The model under review builds one solid part; all positions refer to its coordinate system, in mm. A direction names the side the tool comes from. Round coordinates to 2 decimals unless told otherwise and drop trailing zeros. Loops run counter-clockwise (first coordinate to the right, second up) from the corner with the lowest first, then second, coordinate; pieces in that order, holes last. Notation, with made-up numbers: (48.25, 25) -> (85.25, 25) arc R27 cw to (85.25, 56) -> close; hole circle Ø10 at (-26, -11.75). An arc over 180 degrees is marked (long way). Return JSON: item names as keys, results as strings. Group by question number.
```python
from build123d import *

# Parameters (mm, degrees)
CROQUIS1_W              = 25
CROQUIS1_H              = 28
CROQUIS1_R              = 1.25
CROQUIS1_W_2            = 9.5
CROQUIS1_H_2            = 5
SALIENTE_EXTRUIR1_DEPTH = 1.5
CROQUIS2_W              = 2.5
CROQUIS2_H              = 3
CROQUIS2_W_2            = 5
CORTAR_EXTRUIR1_DEPTH   = 10
REDONDEO1_R             = 15
REDONDEO2_R             = 3


with BuildPart() as part:
    # Croquis1 → Saliente-Extruir1 (new, symmetric)
    with BuildSketch(Plane.XY):
        Rectangle(CROQUIS1_W, CROQUIS1_H)
        with Locations((-10, 4)):
            Circle(CROQUIS1_R, mode=Mode.SUBTRACT)
        with Locations((10, 4)):
            Circle(CROQUIS1_R, mode=Mode.SUBTRACT)
        with Locations((0, 9.2)):
            Rectangle(CROQUIS1_W_2, CROQUIS1_H_2, mode=Mode.SUBTRACT)
    extrude(amount=SALIENTE_EXTRUIR1_DEPTH, both=True)

    # Croquis2 → Cortar-Extruir1 (cut)
    with BuildSketch(Plane.XY.offset(1.5)):
        with Locations((-11.25, -12.5)):
            Rectangle(CROQUIS2_W, CROQUIS2_H)
        with Locations((-7.5, -12.5)):
            Rectangle(CROQUIS2_W_2, CROQUIS2_H)
        with Locations((7.5, -12.5)):
            Rectangle(CROQUIS2_W_2, CROQUIS2_H)
        with Locations((11.25, -12.5)):
            Rectangle(CROQUIS2_W, CROQUIS2_H)
        with BuildLine():
            Line((-12.5, -11), (-10, -11))
            Line((-10, -11), (-10, 1.5))
            ThreePointArc((-10, 1.5), (-11.767766953, 2.232233047), (-12.5, 4))
            Line((-12.5, 4), (-12.5, -11))
        make_face()
        with BuildLine():
            Line((10, 1.5), (10, -11))
            Line((10, -11), (12.5, -11))
            Line((12.5, -11), (12.5, 4))
            ThreePointArc((12.5, 4), (11.767766953, 2.232233047), (10, 1.5))
        make_face()
        with BuildLine():
            Line((12.5, 14), (10, 14))
            Line((10, 14), (10, 6.5))
            ThreePointArc((10, 6.5), (11.767766953, 5.767766953), (12.5, 4))
            Line((12.5, 4), (12.5, 14))
        make_face()
        with BuildLine():
            ThreePointArc((-12.5, 4), (-11.767766953, 5.767766953), (-10, 6.5))
            Line((-10, 6.5), (-10, 14))
            Line((-10, 14), (-12.5, 14))
            Line((-12.5, 14), (-12.5, 4))
        make_face()
    extrude(amount=-CORTAR_EXTRUIR1_DEPTH, mode=Mode.SUBTRACT)

    # Redondeo1
    redondeo1_edges = [part.edges().sort_by_distance(p)[0] for p in [
        (-10, 6.5, 0),
        (-10, 1.5, 0),
        (10, 1.5, 0),
        (10, 6.5, 0),
    ]]
    fillet(redondeo1_edges, radius=REDONDEO1_R)

    # Redondeo2
    redondeo2_edges = [part.edges().sort_by_distance(p)[0] for p in [
        (10, 14, 0),
        (-10, 14, 0),
    ]]
    fillet(redondeo2_edges, radius=REDONDEO2_R)


solid = part.part
```
1. For P1, Ø0.9, axis at y = -13, z = 0.5, coming from the +X side; P2, Ø1.5, axis at y = 9, z = 0.5, coming from the +X side; P3, Ø3, axis at x = 10, y = 4, coming from the -Z side; P4, Ø0.9, axis at y = 8.5, z = 0.5, coming from the -X side, all flat-tipped, find the tip position at first contact; note any pin that passes through.
2. We need section C-C, the plane z = 0.65. Give the number of separate pieces and of enclosed holes in the cut face, then the cut area to 3 significant figures.
3. We need section D-D, the plane y = -10.5. Write out the cut boundary in (x, z), then the cut area to 3 significant figures.
4. Wall thickness on line 1 (Y direction, x = 3.25, z = 1); line 2 (X direction, y = 3.5, z = -0.2); line 3 (X direction, y = 5, z = 0.2): over which ranges is each line inside the solid? List them lowest first.
5. Tool access review of faces 5 (the face through (0, -14, 0)), 6 (the face through (0, 0, 1.5)), 7 (the face through (0, 6.7, 0)), 8 (the face through (10, -8, 0)), 9 (the face through (-10, -8, 0)): name each direction out of +Z, -Z, +X, -X, +Y, -Y from which nothing blocks a thin tool from reaching the whole face with its end or side.
6. We need section A-A, the plane x = 3.75. Write out the cut boundary in (y, z), then the cut area to 3 significant figures.
7. We need section B-B, the plane y = 10. Write out the cut boundary in (x, z).
8. Draft analysis for pull direction X (two halves, no side actions). For faces 1 (the face through (5, -13, 0)), 2 (the face through (-7, -11, 0)), 3 (the face through (4.75, 9, 0)), 4 (the face through (-5, -13, 0)), state which applies: pulls with the +X half, pulls with the -X half, needs draft (parallel to the pull), parting line crosses it, or undercut.
Check sheet entries:
{
 "1": {"P1": "stops at x = 5", "P2": "stops at x = 10.78", "P3": "stops at z = -1.5", "P4": "stops at x = -10.85"},
 "2": {"separate pieces": "1", "enclosed holes": "3", "area": "503 mm²"},
 "3": {"outline": "(-10, -1.5) -> (10, -1.5) -> (10, 1.5) -> (-10, 1.5) -> close", "area": "60.0 mm²"},
 "4": {"line 1": "y = -14 to 6.7, 11.7 to 14", "line 2": "x = -12.45 to -11.15, -8.85 to 8.85, 11.15 to 12.45", "line 3": "x = -12.29 to -10.75, -9.25 to 9.25, 10.75 to 12.29"},
 "5": {"face 5": "+Z, -Z, +X, -X, -Y", "face 6": "+Z, +X, -X, +Y, -Y", "face 7": "+Z, -Z", "face 8": "+Z, -Z, +X, -Y", "face 9": "+Z, -Z, -X, -Y"},
 "6": {"outline": "(-14, -1.5) -> (6.7, -1.5) -> (6.7, 1.5) -> (-14, 1.5) -> close; (11.7, -1.5) -> (14, -1.5) -> (14, 1.5) -> (11.7, 1.5) -> close", "area": "69.0 mm²"},
 "7": {"outline": "(-10.31, -1.5) -> (-4.75, -1.5) -> (-4.75, 1.5) -> (-10.31, 1.5) -> close; (4.75, -1.5) -> (10.31, -1.5) -> (10.31, 1.5) -> (4.75, 1.5) -> close"},
 "8": {"face 1": "pulls with the +X half", "face 2": "needs draft", "face 3": "undercut", "face 4": "pulls with the -X half"}
}
